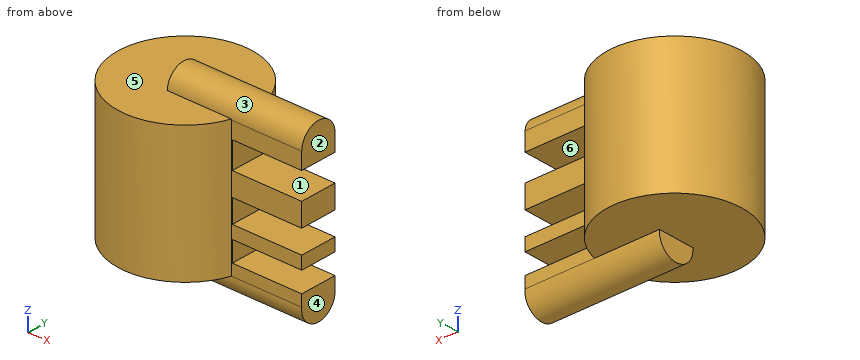
from build123d import *

# Parameters (mm, degrees)
F0_R     = 63.5
F1_DEPTH = 127
F3_DEPTH = 127
F4_W     = 65.542905265
F4_H     = 24.9171182513
F4_H_2   = 21.7300467193
F4_H_3   = 19.1224422306
F5_DEPTH = 35.56


with BuildPart() as f1:
    # F0 (on Top) → F1 (new body)
    with BuildSketch(Plane.XY):
        Circle(F0_R)
    extrude(amount=F1_DEPTH)

    # F2 (on Right) → F3 (join)
    with BuildSketch(Plane.YZ):
        with BuildLine():
            ThreePointArc((15.9773435444, 127.7705729008), (-2.3077528181, 143.6512031965), (-19.0271344036, 126.1297464371))
            Line((-19.0271344036, 126.1297464371), (-19.0271344036, 0))
            ThreePointArc((-19.0271344036, 0), (-1.5248954296, -19.3635171715), (15.9773435444, 0))
            Line((15.9773435444, 0), (15.9773435444, 127.7705729008))
        make_face()
    extrude(amount=F3_DEPTH)

    # F4 (on face) → F5 (cut)
    with BuildSketch(Plane(origin=(0, 15.9773435444, 0), x_dir=(-1, 0, 0), z_dir=(0, 1, 0))):
        with Locations((-94.2285473675, 98.0738960207)):
            Rectangle(F4_W, F4_H)
        with Locations((-94.2285473675, 53.0202630907)):
            Rectangle(F4_W, F4_H_2)
        with Locations((-94.2285473675, 20.4251902178)):
            Rectangle(F4_W, F4_H_3)
    extrude(amount=-F5_DEPTH, mode=Mode.SUBTRACT)


solid = f1.part
Geometry: final body of the model. Coordinates: model frame, mm. Face numbers are marked on the shaded views. A direction names the side the tool comes from. Round coordinates to 2 decimals unless told otherwise and drop trailing zeros. Loops run counter-clockwise (first coordinate to the right, second up) from the corner with the lowest first, then second, coordinate; pieces in that order, holes last. Notation, with made-up numbers: M 7.25,17.5 L 29.25,17.5 A34 ccw 29.25,52.5 Z; hole C 73.25,58.25 d11. An arc over 180 degrees is marked long. Put each result on its own line as item: value. Start each with the question number.
(1) Section query A-A (x = 99). Return loops of the section in (y, z), then the cut area to 3 significant figures.
(2) Draft query along Z for the marked faces 1, 2 and 3. Return one class per face: +Z half, -Z half, draft (parallel to the pull), parting line (faces both ways), or undercut.
(3) Section query C-C (z = 25). Return loops of the section in (x, y), then the cut area to 3 significant figures.
(4) Section query D-D (x = 16). Return loops of the section in (y, z).
(5) Section query B-B (y = -8.5). Return loops of the section in (x, z).
(6) Material intervals for line 1 along Z through (x, y) = (53, -21); line 2 along Y through (x, z) = (90, 120); line 3 along X through (y, z) = (-53, 91) (3 decimals), sorted ascending. Write a range as [from, to].
(7) Set-up query: the marked faces 4, 5 and 6. Return all of +Z, -Z, +X, -X, +Y, -Y with unobstructed straight access to the full face (end or side cutting, diameter ignored); none if empty.
(8) Contact query for flat-ended pins moving along their axis: pin 1 Ø13.5 at (x, z) = (85, 38) entering from +Y; pin 2 Ø3 at (x, y) = (25.5, 9) entering from -Z; pin 3 Ø5 at (y, z) = (4, 138.5) entering from -X. Output: stop coordinate, or through.
Findings below:
1. outline: M -19.03,0 A17.59 ccw long 15.98,0 L 15.98,10.86 L -19.03,10.86 Z; M -19.03,29.99 L 15.98,29.99 L 15.98,42.16 L -19.03,42.16 Z; M -19.03,63.89 L 15.98,63.89 L 15.98,85.62 L -19.03,85.62 Z; M -19.03,110.53 L 15.98,110.53 L 15.98,127.77 A17.54 ccw -19.03,126.13 Z
1. area: 3,140 mm2
2. face 1: undercut
2. face 2: draft
2. face 3: +Z half
3. outline: M 60.58,-19.03 L 61.46,-19.03 L 61.46,15.98 A63.5 ccw long Z
3. area: 12,600 mm2
4. outline: M -61.45,0 L -19.03,0 A17.59 ccw long 15.98,0 L 61.45,0 L 61.45,127 L 15.98,127 L 15.98,127.77 A17.54 ccw -19.01,127 L -61.45,127 Z
5. outline: M -62.93,0 L 0,0 L 0,-17.92 L 127,-17.92 L 127,10.86 L 61.46,10.86 L 61.46,29.99 L 127,29.99 L 127,42.16 L 61.46,42.16 L 61.46,63.89 L 127,63.89 L 127,85.62 L 61.46,85.62 L 61.46,110.53 L 127,110.53 L 127,142.21 L 0,142.21 L 0,127 L -62.93,127 Z
6. line 1: z = [0, 127]
6. line 2: y = [-19.03, 15.98]
6. line 3: x = [-34.975, 34.975]
7. face 4: +Z, -Z, +X, +Y, -Y
7. face 5: +Z, -X
7. face 6: +X, +Y, -Y
8. pin 1: stops at y = 15.98
8. pin 2: stops at z = -16.87
8. pin 3: stops at x = 0
